```python
from build123d import *

# Parameters (mm, degrees)
SKETCH2_R           = 1.5
SKETCH2_R_2         = 4.5
BOSS_EXTRUDE1_DEPTH = 10


with BuildPart() as part:
    # Sketch2 → Boss-Extrude1 (new body)
    with BuildSketch(Plane.XY):
        with BuildLine():
            Line((-56.660710118, 0), (0, 0))
            Line((0, 0), (127.339289882, 0))
            ThreePointArc((127.339289882, 0), (134.410357694, 2.928932188), (137.339289882, 10))
            Line((137.339289882, 10), (137.339289882, 15))
            ThreePointArc((137.339289882, 15), (134.410357694, 22.071067812), (127.339289882, 25))
            Line((127.339289882, 25), (-56.660710118, 25))
            ThreePointArc((-56.660710118, 25), (-63.73177793, 22.071067812), (-66.660710118, 15))
            Line((-66.660710118, 15), (-66.660710118, 10))
            ThreePointArc((-66.660710118, 10), (-63.73177793, 2.928932188), (-56.660710118, 0))
        make_face()
        Polygon((97.839289882, 6.5), (97.839289882, 12.5), (97.839289882, 18.5), (120.839289882, 18.5), (120.839289882, 12.5), (120.839289882, 6.5), align=None, mode=Mode.SUBTRACT)
        with Locations((-56.810710118, 12.5)):
            Circle(SKETCH2_R, mode=Mode.SUBTRACT)
        with Locations((-46.660710118, 12.5)):
            Circle(SKETCH2_R_2, mode=Mode.SUBTRACT)
        with Locations((-36.510710118, 12.5)):
            Circle(SKETCH2_R, mode=Mode.SUBTRACT)
        with BuildLine():
            ThreePointArc((96.099859372, 13.312997269), (96.278187765, 12.923760406), (96.339289882, 12.5))
            ThreePointArc((96.339289882, 12.5), (93.400391999, 12.076239594), (96.099859372, 13.312997269))
        make_face(mode=Mode.SUBTRACT)
        with BuildLine():
            ThreePointArc((125.339289882, 12.5), (123.839289882, 11), (122.339289882, 12.5))
            ThreePointArc((122.339289882, 12.5), (122.373700536, 12.819449323), (122.475353708, 13.124242033))
            ThreePointArc((122.475353708, 13.124242033), (124.158739205, 13.965589346), (125.339289882, 12.5))
        make_face(mode=Mode.SUBTRACT)
    extrude(amount=BOSS_EXTRUDE1_DEPTH)


solid = part.part
```
Source: CAD feature listing. Evaluate the final solid. Frame: model axes, mm. A direction names the side the tool comes from. Coordinates: 2 decimals unless noted, no trailing zeros. Loops run counter-clockwise (first coordinate to the right, second up) from the corner with the lowest first, then second, coordinate; pieces in that order, holes last. Notation, with made-up numbers: (19.5, 57.5) -> (78.5, 57.5) arc R21 ccw to (78.5, 61.5) -> close; hole circle Ø9 at (65, -26.75). An arc over 180 degrees is marked (long way). One line per item, written item: value. Start each with the question number.
Q1. Contact query for a flat-ended pin moving along its axis: P1, Ø1, axis at y = 18, z = 2, coming from the -X side. Output: stop coordinate, or through.
Q2. Section query A-A, the plane x = 117.5. Return the cut outline in (y, z), and give its area (3 significant figures).
Q3. Mould query, pull axis Y, two halves, no side actions, for faces 1 (the face through (34, 13, 0)), 2 (the face through (134.49, 21.99, 4.93)), 3 (the face through (97.839, 12, 5)), 4 (the face through (-42.37, 13.85, 4.93)). Classes: pulls with the +Y half, pulls with the -Y half, needs draft (parallel to the pull), parting line crosses it, or undercut.
Q4. Section query C-C, the plane y = 23. Return the cut outline in (x, z).
Q5. Section query B-B, the plane z = 4. Return the cut outline in (x, y).
Q6. Set-up query: faces 5 (the face through (-66.661, 13, 5)), 6 (the face through (120.839, 13, 5)). Return all of +Z, -Z, +X, -X, +Y, -Y with unobstructed straight access to the full face (end or side cutting, diameter ignored); none if empty.
Q7. Line query: line 1 along Y through (x, z) = (104, 6.5); line 2 along X through (y, z) = (17.5, 8); line 3 along X through (y, z) = (7.75, 1.25). Output: solid intervals per line, ascending.
Results:
1. P1: x = -66.34
2. outline: (0, 0) -> (6.5, 0) -> (6.5, 10) -> (0, 10) -> close; (18.5, 0) -> (25, 0) -> (25, 10) -> (18.5, 10) -> close
2. area: 130 mm^2
3. face 1: needs draft
3. face 2: pulls with the +Y half
3. face 3: undercut
3. face 4: undercut
4. outline: (-62.66, 0) -> (133.34, 0) -> (133.34, 10) -> (-62.66, 10) -> close
5. outline: (-66.66, 10) arc R10 ccw to (-56.66, 0) -> (127.34, 0) arc R10 ccw to (137.34, 10) -> (137.34, 15) arc R10 ccw to (127.34, 25) -> (-56.66, 25) arc R10 ccw to (-66.66, 15) -> close; hole circle Ø3 at (-56.81, 12.5); hole circle Ø9 at (-46.66, 12.5); hole circle Ø3 at (-36.51, 12.5); hole circle Ø3 at (94.84, 12.5); hole (97.84, 6.5) -> (120.84, 6.5) -> (120.84, 18.5) -> (97.84, 18.5) -> close; hole circle Ø3 at (123.84, 12.5)
6. face 5: +Z, -Z, -X, +Y, -Y
6. face 6: +Z, -Z
7. line 1: 0 to 6.5, 18.5 to 25
7. line 2: -66.34 to 97.84, 120.84 to 137.02
7. line 3: -66.4 to 97.84, 120.84 to 137.08
